The model under review builds one solid part; all positions refer to its coordinate system, in mm. Round coordinates to 2 decimals unless told otherwise and drop trailing zeros. Order: outer loops, then holes, each group sorted by start corner. A loop starts at its lowest first (then second) coordinate and runs counter-clockwise, first axis right, second up.
Autodesk Fusion 360 part; units mm, degrees
sketch "Sketch1" plane through (0, 0, 0) normal (0, 0, 1) x (1, 0, 0)
  line L0 (0, 0) -> (60, 0)
  line L1 (30, 0) -> (30, -130)
  line L2 (30, -130) -> (75, -130)
  line L3 (30, -130) -> (-15, -130)
  line L4 (0, 0) -> (-15, -130)
  line L5 (60, 0) -> (75, -130)
  dimension "d1" = 60
  dimension "d2" = 130
  dimension "d3" = 45
  dimension "d4" = 45
extrude "Extrude1" add sketch "Sketch1" along normal blind 2
sketch "Sketch2" plane through (0, 0, 2) normal (0, 0, 1) x (-1, 0, 0)
  line L0 (0, 0) -> (15, 130)
  line L1 (15, 130) -> (-75, 130)
  line L2 (-75, 130) -> (-60, 0)
  line L3 (-60, 0) -> (0, 0)
  line L4 (-30, 0) -> (-30, 3.5)
  line L5 (-60, 0) -> (-50, 0)
  line L6 (-50, 0) -> (-50, 3.5)
  line L7 (-30, 0) -> (-30, 130)
  line L8 (-62.991, 25.9222) -> (-59.5141, 26.3233)
  line L9 (-64.2385, 36.7338) -> (-60.7616, 37.135)
  line L10 (-59.5141, 26.3233) -> (-71.4768, 130)
  line L11 (-60.7616, 37.135) -> (-56.4649, 0)
  line L12 (-60.7616, 37.135) -> (-23.3789, 37.135) construction
  line L13 (-71.4768, 130) -> (-70.5598, 122.0527)
  line L14 (-70.5598, 122.0527) -> (-67.1211, 92.2505)
  line L15 (-67.1211, 92.2505) -> (-63.6823, 62.4482)
  line L16 (-63.6823, 62.4482) -> (-60.2436, 32.6459)
  line L17 (-60.2436, 32.6459) -> (-57.9511, 12.7777)
  point P0 (11.4768, 130)
  point P1 (10.5598, 122.0527)
  point P2 (7.1211, 92.2505)
  point P3 (3.6823, 62.4482)
  point P4 (0.2436, 32.6459)
  point P5 (-2.0489, 12.7777)
  point P6 (-10, 3.5)
  dimension "d7" = 3.5
  dimension "d8" = 10
  dimension "d9" = 3.5
  dimension "d10" = 3.5
  dimension "d11" = 3.5
  dimension "d12" = 83.4
  dimension "d13" = 8
  dimension "d14" = 30
  dimension "d15" = 30
  dimension "d16" = 30
  dimension "d17" = 20
hole "Hole1" at (10, -3.5, 2) at (2.0489, -12.7777, 2) at (-0.2436, -32.6459, 2) at (-3.6823, -62.4482, 2) at (-7.1211, -92.2505, 2) at (-10.5598, -122.0527, 2) at (50, -3.5, 2) at (57.9511, -12.7777, 2) at (63.6823, -62.4482, 2) at (67.1211, -92.2505, 2) at (70.5598, -122.0527, 2) at (60.2436, -32.6459, 2) direction (0, 0, -1) diameter 4 depth 50 tip angle 180
(1) Clearance check with a flat-ended pin moving along its axis: P1, Ø4.5, axis at x = 63.68, y = -62.45, coming from the +Z side. State where the tip first meets the part, or that it passes through.
(2) We need section D-D (y = -112.5). Give the boundary of the cut face in (x, z).
(3) The part is to be moulded in two halves that separate along X. For faces 1 (the flat face through (-7.395, -64.09, 0.986)), 2 (the cylindrical face through (69.208, -120.579, 0.986)), 3 (the flat face through (29, -64, 2)), 4 (the cylindrical face through (0.522, -34.493, 0.986)), say which applies: pulls with the +X half, pulls with the -X half, needs draft (parallel to the pull), parting line crosses it, or undercut.
(4) We need section A-A (x = 10). Give the boundary of the cut face in (y, z).
(5) We need section B-B (y = -3.5). Give the boundary of the cut face in (x, z), and give its area (3 significant figures).
(6) To check wall thickness, follow L1, parallel to Y at x = 50, z = 0.75; L2, parallel to X at y = -3.5, z = 0.7; L3, parallel to Y at x = 3.5, z = 0.95. State the ranges of each line that lie inside material, in increasing order.
(7) We need section C-C (z = 1.65). Count the separate pieces of the cut face and the enclosed holes in it, and give its area (3 significant figures).
Verdict:
1. P1: stops at z = 2
2. outline: (-12.98, 0) - (72.98, 0) - (72.98, 2) - (-12.98, 2) - close
3. face 1: pulls with the -X half
3. face 2: undercut
3. face 3: needs draft
3. face 4: undercut
4. outline: (-130, 0) - (-5.5, 0) - (-5.5, 2) - (-130, 2) - close; (-1.5, 0) - (0, 0) - (0, 2) - (-1.5, 2) - close
5. outline: (-0.4, 0) - (8, 0) - (8, 2) - (-0.4, 2) - close; (12, 0) - (48, 0) - (48, 2) - (12, 2) - close; (52, 0) - (60.4, 0) - (60.4, 2) - (52, 2) - close
5. area: 106 mm2
6. L1: y = -130 to -5.5, -1.5 to 0
6. L2: x = -0.4 to 8, 12 to 48, 52 to 60.4
6. L3: y = -130 to -14.15, -11.4 to 0
7. separate pieces: 1
7. enclosed holes: 12
7. area: 9,600 mm2
